from build123d import *

# Parameters (mm, degrees)
CROQUIS2_R              = 50
SALIENTE_EXTRUIR2_DEPTH = 3
SALIENTE_EXTRUIR3_START = 1
CROQUIS3_R              = 50
SALIENTE_EXTRUIR3_DEPTH = 1
CROQUIS4_R              = 18
SALIENTE_EXTRUIR4_DEPTH = 6
CROQUIS5_R              = 50
CROQUIS5_R_2            = 49
SALIENTE_EXTRUIR5_DEPTH = 0.5
SALIENTE_EXTRUIR6_DEPTH = 2
SALIENTE_EXTRUIR7_DEPTH = 2


with BuildPart() as part:
    # Croquis2 → Saliente-Extruir2 (new body)
    with BuildSketch(Plane(origin=(0, 0, -5), x_dir=(-1, 0, 0), z_dir=(0, 0, -1))):
        Circle(CROQUIS2_R)
        with BuildLine():
            Line((-26.088038734, 4.654485475), (-31.293290297, 2.702516138))
            ThreePointArc((-31.293290297, 2.702516138), (-40.5, 0), (-31.293290297, -2.702516138))
            Line((-31.293290297, -2.702516138), (-26.088038734, -4.654485475))
            ThreePointArc((-26.088038734, -4.654485475), (-18.738329701, -18.738329701), (-4.654485475, -26.088038734))
            Line((-4.654485475, -26.088038734), (-2.702516138, -31.293290297))
            ThreePointArc((-2.702516138, -31.293290297), (0, -40.5), (2.702516138, -31.293290297))
            Line((2.702516138, -31.293290297), (4.654485475, -26.088038734))
            ThreePointArc((4.654485475, -26.088038734), (18.738329701, -18.738329701), (26.088038734, -4.654485475))
            Line((26.088038734, -4.654485475), (31.293290297, -2.702516138))
            ThreePointArc((31.293290297, -2.702516138), (40.5, 0), (31.293290297, 2.702516138))
            Line((31.293290297, 2.702516138), (26.088038734, 4.654485475))
            ThreePointArc((26.088038734, 4.654485475), (18.738329701, 18.738329701), (4.654485475, 26.088038734))
            Line((4.654485475, 26.088038734), (2.702516138, 31.293290297))
            ThreePointArc((2.702516138, 31.293290297), (0, 40.5), (-2.702516138, 31.293290297))
            Line((-2.702516138, 31.293290297), (-4.654485475, 26.088038734))
            ThreePointArc((-4.654485475, 26.088038734), (-18.738329701, 18.738329701), (-26.088038734, 4.654485475))
        make_face(mode=Mode.SUBTRACT)
    extrude(amount=-SALIENTE_EXTRUIR2_DEPTH)

    # Croquis3 → Saliente-Extruir3 (add)
    with BuildSketch(Plane(origin=(0, 0, -5), x_dir=(-1, 0, 0), z_dir=(0, 0, -1)).offset(SALIENTE_EXTRUIR3_START)):
        Circle(CROQUIS3_R)
    extrude(amount=-SALIENTE_EXTRUIR3_DEPTH)

    # Croquis4 → Saliente-Extruir4 (add)
    with BuildSketch(Plane(origin=(0, 0, -6), x_dir=(-1, 0, 0), z_dir=(0, 0, -1))):
        Circle(CROQUIS4_R)
    extrude(amount=SALIENTE_EXTRUIR4_DEPTH)

    # Croquis5 → Saliente-Extruir5 (add)
    # profile 1 of 5: a face of its own
    with BuildSketch(Plane.XY.offset(-2)):
        with Locations(Location((0, 0, 0), (0, 0, 180))):
            Circle(CROQUIS5_R)
        Circle(CROQUIS5_R_2, mode=Mode.SUBTRACT)
    # profile 2 of 5: a face of its own
    with BuildSketch(Plane.XY.offset(-2)):
        with BuildLine():
            Line((-30.425241187, 28.617399842), (-23.823505496, 22.01566415))
            ThreePointArc((-23.823505496, 22.01566415), (-22.01566415, 22.01566415), (-22.01566415, 23.823505496))
            Line((-22.01566415, 23.823505496), (-28.617399842, 30.425241187))
            ThreePointArc((-28.617399842, 30.425241187), (-30.425241187, 30.425241187), (-30.425241187, 28.617399842))
        make_face()
    # profile 3 of 5: a face of its own
    with BuildSketch(Plane.XY.offset(-2)):
        with BuildLine():
            Line((30.425241187, -28.617399842), (23.823505496, -22.01566415))
            ThreePointArc((23.823505496, -22.01566415), (22.01566415, -22.01566415), (22.01566415, -23.823505496))
            Line((22.01566415, -23.823505496), (28.617399842, -30.425241187))
            ThreePointArc((28.617399842, -30.425241187), (30.425241187, -30.425241187), (30.425241187, -28.617399842))
        make_face()
    # profile 4 of 5: a face of its own
    with BuildSketch(Plane.XY.offset(-2)):
        with BuildLine():
            Line((-28.617399842, -30.425241187), (-22.01566415, -23.823505496))
            ThreePointArc((-22.01566415, -23.823505496), (-22.01566415, -22.01566415), (-23.823505496, -22.01566415))
            Line((-23.823505496, -22.01566415), (-30.425241187, -28.617399842))
            ThreePointArc((-30.425241187, -28.617399842), (-30.425241187, -30.425241187), (-28.617399842, -30.425241187))
        make_face()
    # profile 5 of 5: a face of its own
    with BuildSketch(Plane.XY.offset(-2)):
        with BuildLine():
            Line((28.617399842, 30.425241187), (22.01566415, 23.823505496))
            ThreePointArc((22.01566415, 23.823505496), (22.01566415, 22.01566415), (23.823505496, 22.01566415))
            Line((23.823505496, 22.01566415), (30.425241187, 28.617399842))
            ThreePointArc((30.425241187, 28.617399842), (30.425241187, 30.425241187), (28.617399842, 30.425241187))
        make_face()
    extrude(amount=SALIENTE_EXTRUIR5_DEPTH)

    # Croquis6 → Saliente-Extruir6 (add)
    with BuildSketch(Plane(origin=(0, 0, -6), x_dir=(-1, 0, 0), z_dir=(0, 0, -1))):
        Polygon((-30.318233872, -37.389301684), (-35.355339059, -42.426406871), (-42.426406871, -35.355339059), (-38.890872965, -31.819805153), (-37.389301684, -30.318233872), align=None)
    extrude(amount=-SALIENTE_EXTRUIR6_DEPTH)

    # Croquis7 → Saliente-Extruir7 (add)
    with BuildSketch(Plane(origin=(0, 0, -6), x_dir=(-1, 0, 0), z_dir=(0, 0, -1))):
        Polygon((-42.426406871, -35.355339059), (-41.014653165, -33.943585354), (-33.943585354, -41.014653165), (-35.355339059, -42.426406871), align=None)
    extrude(amount=SALIENTE_EXTRUIR7_DEPTH)


solid = part.part
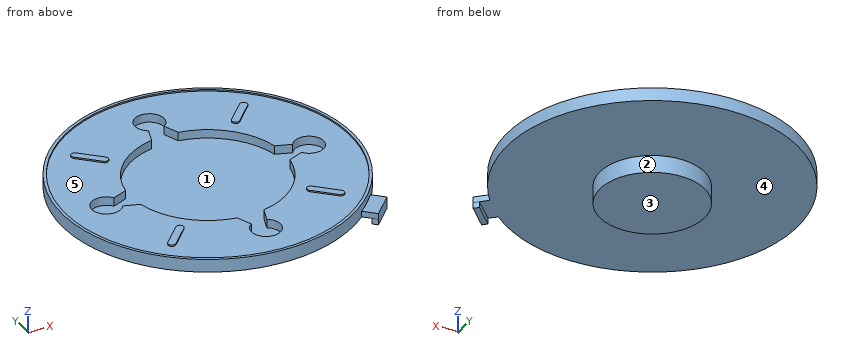
Source: CAD feature listing. Evaluate the final solid. Frame: model axes, mm. Face numbers are marked on the shaded views. A direction names the side the tool comes from. Coordinates: 2 decimals unless noted, no trailing zeros. Loops run counter-clockwise (first coordinate to the right, second up) from the corner with the lowest first, then second, coordinate; pieces in that order, holes last. Notation, with made-up numbers: (77.5, 59.5) - (118.5, 59.5) arc R22 cw to (118.5, 84.5) - close; hole circle Ø1 at (-38.5, 82). An arc over 180 degrees is marked (long way). One line per item, written item: value. Start each with the question number.
1. Contact query for flat-ended pins moving along their axis: P1, Ø4, axis at y = 23, z = -3.5, coming from the +X side; P2, Ø13, axis at x = -35.5, y = 0, coming from the -Z side; P3, Ø1, axis at x = -16.5, y = -5, coming from the +Z side. Output: stop coordinate, or through.
2. Section A-A (y = 0). Return the cut outline in (x, z), and give its area (3 significant figures).
3. Section C-C (z = -10.5). Return the cut outline in (x, y), and give its area (3 significant figures).
4. Set-up query: the marked faces 4 and 5. Return all of +Z, -Z, +X, -X, +Y, -Y with unobstructed straight access to the full face (end or side cutting, diameter ignored); none if empty.
5. Section D-D (x = -35.5). Return the cut outline in (y, z) (3 decimals).
6. Mould query, pull axis X, two halves, no side actions, for the marked faces 1, 2 and 3. Classes: pulls with the +X half, pulls with the -X half, needs draft (parallel to the pull), parting line crosses it, or undercut.
7. Ray query, L1, parallel to Z at x = -33.5, y = 15.5; L2, parallel to Z at x = 0, y = -15; L3, parallel to Y at x = 0, z = -1.75. Return the intervals inside material, ascending.
Verdict:
1. P1: stops at x = 45.38
1. P2: stops at z = -6
1. P3: stops at z = -5
2. outline: (-50, -6) - (-18, -6) - (-18, -12) - (18, -12) - (18, -6) - (50, -6) - (50, -1.5) - (49, -1.5) - (49, -2) - (40.5, -2) - (40.5, -5) - (-40.5, -5) - (-40.5, -2) - (-49, -2) - (-49, -1.5) - (-50, -1.5) - close
2. area: 374 mm2
3. outline: circle Ø36 at (0, 0)
3. area: 1,020 mm2
4. face 4: -Z
4. face 5: +Z
5. outline: (-35.21, -6) - (35.21, -6) - (35.21, -1.5) - (33.775, -1.5) - (33.775, -2) - (5, -2) - (5, -5) - (-5, -5) - (-5, -2) - (-33.775, -2) - (-33.775, -1.5) - (-35.21, -1.5) - close
6. face 1: undercut
6. face 2: parting line crosses it
6. face 3: needs draft
7. L1: z = -6 to -2
7. L2: z = -12 to -5
7. L3: y = -50 to -49, 49 to 50
